Verification items for the finished model (mm, model axes). Give positions to 0.01 mm unless a question says otherwise; leave off trailing zeros. Loops run counter-clockwise (first coordinate to the right, second up) from the corner with the lowest first, then second, coordinate; pieces in that order, holes last. Notation, with made-up numbers: (56, -32.75) - (111, -32.75) arc R10 ccw to (111, -19.75) - close; hole circle Ø4 at (42.25, 1.25). An arc over 180 degrees is marked (long way). Use one line per item in the form item = value.
```python
from build123d import *

# Parameters (mm, degrees)
F0_W     = 16
F0_H     = 16
F1_DEPTH = 18
F2_W     = 31.5
F2_H     = 27
F2_W_2   = 16
F2_H_2   = 16
F3_DEPTH = 277
F4_R     = 8
F5_DEPTH = 23
F6_R     = 3
F7_DEPTH = 25


with BuildPart() as f1:
    # F0 (on Top) → F1 (new body)
    with BuildSketch(Plane.XY):
        Rectangle(F0_W, F0_H)
    extrude(amount=F1_DEPTH)

    # F2 (on face) → F3 (join)
    with BuildSketch(Plane.XY.offset(18)):
        with Locations((-1.75, 0)):
            Rectangle(F2_W, F2_H)
        Rectangle(F2_W_2, F2_H_2, mode=Mode.SUBTRACT)
        Rectangle(F2_W_2, F2_H_2)
    extrude(amount=F3_DEPTH)

    # F4 (on face) → F5 (join)
    with BuildSketch(Plane.XY.offset(295)):
        with Locations((1, 0)):
            Circle(F4_R)
    extrude(amount=F5_DEPTH)

    # F6 (on face) → F7 (cut)
    with BuildSketch(Plane(origin=(0, 13.5, 0), x_dir=(-1, 0, 0), z_dir=(0, 1, 0))):
        with Locations((0, 8)):
            Circle(F6_R)
        with Locations((0, 310)):
            Circle(F6_R)
    extrude(amount=-F7_DEPTH, mode=Mode.SUBTRACT)


solid = f1.part
```
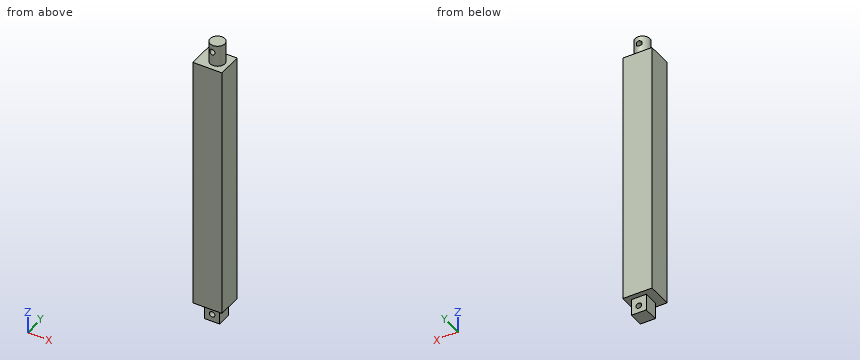
1. Section check B-B, the plane y = 0. Record the cut outline in (x, z), then the cut area to 3 significant figures.
Result set:
outline = (-17.5, 18) - (-8, 18) - (-8, 0) - (8, 0) - (8, 18) - (14, 18) - (14, 295) - (9, 295) - (9, 318) - (-7, 318) - (-7, 295) - (-17.5, 295) - close; hole circle Ø6 at (0, 8); hole circle Ø6 at (0, 310)
area = 9,320 mm²
2. Section check C-C, the plane x = 0. Record the cut outline in (y, z), then the cut area to 3 significant figures.
Result set:
outline = (-13.5, 18) - (-8, 18) - (-8, 11) - (8, 11) - (8, 18) - (13.5, 18) - (13.5, 295) - (7.94, 295) - (7.94, 307) - (-7.94, 307) - (-7.94, 295) - (-13.5, 295) - close; (-8, 0) - (8, 0) - (8, 5) - (-8, 5) - close; (-7.94, 313) - (7.94, 313) - (7.94, 318) - (-7.94, 318) - close
area = 7,940 mm²
3. Depth check by flat-ended pin: pin 1 Ø13 at (x, z) = (-3.5, 6) entering from -Y; pin 2 Ø5 at (x, z) = (-3, 5) entering from +Y; pin 3 Ø5 at (y, z) = (-3, 11.5) entering from -X. Enter the tip coordinate at first touch or a pass-through.
Result set:
pin_1 = -8
pin_2 = 8
pin_3 = -8
4. Scan lines: probe 1 along Z at (x, y) = (0, 1.5); probe 2 along Z at (x, y) = (-11, 8); probe 3 along X at (y, z) = (-3, 310). Record each from-to range of solid material in increasing order.
Result set:
probe_1 = 0 to 5, 11 to 307, 313 to 318
probe_2 = 18 to 295
probe_3 = -6.42 to -3, 3 to 8.42
5. Section check D-D, the plane z = 310. Record the cut outline in (x, y).
Result set:
outline = (-3, -6.93) - (-3, 6.93) arc R8 ccw to start; (3, -7.75) arc R8 ccw to (3, 7.75) - close
6. Section check A-A, the plane z = 8. Record the cut outline in (x, y), then the cut area to 3 significant figures.
Result set:
outline = (-8, -8) - (-3, -8) - (-3, 8) - (-8, 8) - close; (3, -8) - (8, -8) - (8, 8) - (3, 8) - close
area = 160 mm²
